Design review of the part built by this model. Coordinates are the model's own, in mm. A direction names the side the tool comes from. Round coordinates to 2 decimals unless told otherwise and drop trailing zeros. Order: outer loops, then holes, each group sorted by start corner. A loop starts at its lowest first (then second) coordinate and runs counter-clockwise, first axis right, second up.
from build123d import *

# Parameters (mm, degrees)
BOSS_EXTRU_1_DEPTH      = 7
ESQUISSE2_R             = 3
ENL_V_MAT_EXTRU_1_DEPTH = 7
ESQUISSE3_R             = 1.5
ENL_V_MAT_EXTRU_2_DEPTH = 7
ESQUISSE5_R             = 12.5
ENL_V_MAT_EXTRU_5_DEPTH = 5
ESQUISSE10_W            = 27
ESQUISSE10_H            = 3.5
ENL_V_MAT_EXTRU_6_DEPTH = 20
ESQUISSE12_R            = 6
BOSS_EXTRU_3_DEPTH      = 3.5
ESQUISSE13_R            = 4
ENL_V_MAT_EXTRU_7_DEPTH = 66.295482233
ENL_V_MAT_EXTRU_8_DEPTH = 3.5
BOSS_EXTRU_4_DEPTH      = 4
ESQUISSE16_R            = 6
ESQUISSE16_R_2          = 4
BOSS_EXTRU_5_DEPTH      = 3.5


with BuildPart() as part:
    # Esquisse1 → Boss.-Extru.1 (new body)
    with BuildSketch(Plane.XY):
        with BuildLine():
            Line((8, 0), (13.5, -50))
            ThreePointArc((13.5, -50), (0, -63.5), (-13.5, -50))
            Line((-13.5, -50), (-8, 0))
            ThreePointArc((-8, 0), (0, 8), (8, 0))
        make_face()
    extrude(amount=BOSS_EXTRU_1_DEPTH)

    # Esquisse2 → Enlèv. mat.-Extru.1 (cut)
    with BuildSketch(Plane.XY.offset(7)):
        with Locations((0, -50)):
            Circle(ESQUISSE2_R)
    extrude(amount=-ENL_V_MAT_EXTRU_1_DEPTH, mode=Mode.SUBTRACT)

    # Esquisse3 → Enlèv. mat.-Extru.2 (cut)
    with BuildSketch(Plane.XY.offset(7)):
        with Locations((0, -41)):
            Circle(ESQUISSE3_R)
        with Locations((-7.794228634, -54.5)):
            Circle(ESQUISSE3_R)
        with Locations((7.794228634, -54.5)):
            Circle(ESQUISSE3_R)
    extrude(amount=-ENL_V_MAT_EXTRU_2_DEPTH, mode=Mode.SUBTRACT)

    # Esquisse5 → Enlèv. mat.-Extru.5 (cut)
    with BuildSketch(Plane.XY.offset(7)):
        with Locations((0, -50)):
            Circle(ESQUISSE5_R)
    extrude(amount=-ENL_V_MAT_EXTRU_5_DEPTH, mode=Mode.SUBTRACT)

    # Esquisse10 → Enlèv. mat.-Extru.6 (cut)
    with BuildSketch(Plane(origin=(0, 10, 0), x_dir=(1, 0, 0), z_dir=(0, 1, 0))):
        with Locations((0, -5.25)):
            Rectangle(ESQUISSE10_W, ESQUISSE10_H)
    extrude(amount=-ENL_V_MAT_EXTRU_6_DEPTH, mode=Mode.SUBTRACT)

    # Esquisse12 → Boss.-Extru.3 (add)
    with BuildSketch(Plane.XY.offset(3.5)):
        with Locations(Location((0, 0, 0), (0, 0, 180))):
            Circle(ESQUISSE12_R)
    extrude(amount=BOSS_EXTRU_3_DEPTH)

    # Esquisse13 → Enlèv. mat.-Extru.7 (cut, through all)
    with BuildSketch(Plane.XY.offset(7)):
        Circle(ESQUISSE13_R)
    extrude(amount=-ENL_V_MAT_EXTRU_7_DEPTH, mode=Mode.SUBTRACT)

    # Esquisse14 → Enlèv. mat.-Extru.8 (cut)
    with BuildSketch(Plane.XY.offset(7)):
        Polygon((-9.1, -10), (-10.193404792, -19.940043559), (9.756042875, -15.964026136), (9.1, -10), align=None)
    extrude(amount=-ENL_V_MAT_EXTRU_8_DEPTH, mode=Mode.SUBTRACT)

    # Esquisse15 → Boss.-Extru.4 (add)
    with BuildSketch(Plane.XY.offset(7)):
        Polygon((-10.193404792, -19.940043559), (9.756042875, -15.964026136), (10.630766708, -23.916060983), (-11.068128625, -27.892078407), align=None)
    extrude(amount=BOSS_EXTRU_4_DEPTH)

    # Esquisse16 → Boss.-Extru.5 (add)
    with BuildSketch(Plane(origin=(0, 0, 0), x_dir=(-1, 0, 0), z_dir=(0, 0, -1))):
        Circle(ESQUISSE16_R)
        with Locations(Location((0, 0, 0), (0, 0, 180))):
            Circle(ESQUISSE16_R_2, mode=Mode.SUBTRACT)
    extrude(amount=BOSS_EXTRU_5_DEPTH)


solid = part.part
1) Clearance check with flat-ended pins moving along their axes: P1, Ø7.5, axis at x = 1.5, y = -50.5, coming from the +Z side; P2, Ø2, axis at x = 9.5, z = 4, coming from the -Y side; P3, Ø6, axis at x = -2, y = -0.5, coming from the +Z side. State where each tip first meets the part, or that it passes through.
Results:
P1: stops at z = 2
P2: stops at y = -60.49
P3: stops at z = 7
2) To check wall thickness, follow line 1 along Y through (x, z) = (0, 3); line 2 along Y through (x, z) = (0, 0.9); line 3 along Y through (x, z) = (0.25, 5.25). State the ranges of each line that lie inside material, in increasing order.
Results:
line 1: y = -63.5 to -62.5, -37.5 to -4, 4 to 8
line 2: y = -63.5 to -53, -47 to -42.5, -39.5 to -4, 4 to 8
line 3: y = -63.5 to -62.5, -37.5 to -17.86, -5.99 to -3.99, 3.99 to 5.99
3) Take a section at B-B on x = 0. State how many separate pieces and enclosed holes the cut face has, plus the area to 3 significant figures.
Results:
separate pieces: 4
enclosed holes: 0
area: 299 mm2
4) Take a section at A-A on y = -54.5. Give the boundary of the cut face in (x, z).
Results:
outline: (-12.73, 0) - (-9.29, 0) - (-9.29, 2) - (-11.66, 2) - (-11.66, 7) - (-12.73, 7) - close; (-6.29, 0) - (6.29, 0) - (6.29, 2) - (-6.29, 2) - close; (9.29, 0) - (12.73, 0) - (12.73, 7) - (11.66, 7) - (11.66, 2) - (9.29, 2) - close
5) For faces 5 (the face through (-3.92, -1.42, 7)), 6 (the face through (-2.71, -62.203, 4.535)), 7 (the face through (-0.36, -17.98, 7.2)), 8 (the face through (0.297, -63.497, 3.451)), 9 (the face through (-0.867, 3.905, 1.824)), list the 3-axis set-ups (+Z, -Z, +X, -X, +Y, -Y) from which the entire face can be reached by the end or side of a thin tool; tool diameter is ignored.
Results:
face 5: +Z, +X, -X, +Y
face 6: +Z
face 7: +Z, -X
face 8: +Z, -Z, -Y
face 9: +Z, -Z
6) The part is to be moulded in two halves that separate along Y. For faces 1 (the face through (-0.067, -25.876, 8.972)), 2 (the face through (0, -36, 7)), 3 (the face through (-5.723, -1.802, 5.226)), 4 (the face through (-7.1, -55.83, 1.01)), say which applies: released by +Y, released by -Y, zero draft, split by the parting line, or undercut.
Results:
face 1: released by -Y
face 2: zero draft
face 3: undercut
face 4: undercut
7) Take a section at D-D on x = 4.75. Give the boundary of the cut face in (y, z).
Results:
outline: (-62.64, 0) - (-3.67, 0) - (-3.67, -3.5) - (3.67, -3.5) - (3.67, 0) - (6.44, 0) - (6.44, 3.5) - (3.67, 3.5) - (3.67, 7) - (-3.67, 7) - (-3.67, 3.5) - (-16.96, 3.5) - (-16.96, 11) - (-24.99, 11) - (-24.99, 7) - (-38.44, 7) - (-38.44, 2) - (-61.56, 2) - (-61.56, 7) - (-62.64, 7) - close
8) Take a section at C-C on z = 10. Give the boundary of the cut face in (x, y).
Results:
outline: (-11.07, -27.89) - (10.63, -23.92) - (9.76, -15.96) - (-10.19, -19.94) - close
